Autodesk Inventor part; units mm, degrees
ref_plane "YZ Plane" through (0, 0, 0) normal (1, 0, 0) x (0, 1, 0)
ref_plane "XZ Plane" through (0, 0, 0) normal (0, 1, 0) x (-1, 0, 0)
ref_plane "XY Plane" through (0, 0, 0) normal (0, 0, 1) x (1, 0, 0)
sketch "Sketch1" plane through (0, 0, 0) normal (0, 1, 0) x (-1, 0, 0)
  circle A0 centre (0, 0) radius 2
  dimension "d0" = 4
extrude "Extrusion1" add sketch "Sketch1" along normal blind 12.506
sketch "Sketch2" plane through (0, 12.506, 0) normal (0, 1, 0) x (1, 0, 0)
  circle A0 centre (0, 0) radius 3
  dimension "d3" = 6
extrude "Extrusion2" add sketch "Sketch2" along normal blind 2.445
sketch "Sketch3" plane through (0, 14.951, 0) normal (0, 1, 0) x (1, 0, 0)
  circle A0 centre (0, 0) radius 2
  line L0 (0, 2) -> (1.7321, 1)
  line L1 (1.7321, 1) -> (1.7321, -1)
  line L2 (1.7321, -1) -> (0, -2)
  line L3 (0, -2) -> (-1.7321, -1)
  line L4 (-1.7321, -1) -> (-1.7321, 1)
  line L5 (-1.7321, 1) -> (0, 2)
extrude "Extrusion3" cut sketch "Sketch3" against normal blind 1.5 contours L1 L2 L3 L4 L5 L0
thread "Thread1"
properties part number "4mm_0.5_Screw"
Geometry: final body of the model. Coordinates: model frame, mm. A direction names the side the tool comes from. Coordinates: 2 decimals unless noted, no trailing zeros. Order: outer loops, then holes, each group sorted by start corner. A loop starts at its lowest first (then second) coordinate and runs counter-clockwise, first axis right, second up. Notation, with made-up numbers: M 66.5,82 L 90.5,82 A19 cw 90.5,111 Z; hole C 12.5,27.25 d4. An arc over 180 degrees is marked long. Answer in a Markdown table with one row per item. Add a question column.
Q1. Section query A-A on z = 0. Return the cut outline in (x, y), and give its area (3 significant figures).
Q2. Section query C-C on y = 10.25. Return the cut outline in (x, z).
Q3. Reachability of faces 1 (the flat face through (-0.88, 14.21, -1.49)), 2 (the flat face through (2, 14.951, 0)), 3 (the flat face through (1, 12.506, 2)) from +Z, -Z, +X, -X, +Y, -Y: full face, straight path, thin tool, end or side. Return the list, or none.
Q4. Section query D-D on z = -2.2. Return the cut outline in (x, y), and give its area (3 significant figures).
Q5. Mould query, pull axis Z, two halves, no side actions, for faces 4 (the cylindrical face through (-3, 14, 0)), 5 (the flat face through (0, 0, 0)), 6 (the flat face through (0, 13.451, 0)). Classes: released by +Z, released by -Z, zero draft, split by the parting line, or undercut.
Q6. Contact query for flat-ended pins moving along their axis: P1, Ø2, axis at y = 5, z = 1.5, coming from the -X side; P2, Ø1, axis at x = 1.5, y = 6, coming from the +Z side. Output: stop coordinate, or through.
Q7. Line query: L1, parallel to Y at x = 0.9, z = 0; L2, parallel to Z at x = 0, y = 2; L3, parallel to Y at x = -2.8, z = 0. Output: solid intervals per line, ascending.
Q8. Section query B-B on x = -0.5. Return the cut outline in (y, z), and give its area (3 significant figures).
Completed:
| question | item | result |
|---|---|---|
| 1 | outline | M -3,12.51 L -2,12.51 L -2,0 L 2,0 L 2,12.51 L 3,12.51 L 3,14.95 L 1.73,14.95 L 1.73,13.45 L -1.73,13.45 L -1.73,14.95 L -3,14.95 Z |
| 1 | area | 59.5 mm2 |
| 2 | outline | C 0,0 d4 |
| 3 | face 1 | +Y |
| 3 | face 2 | +Z, -Z, +X, -X, +Y |
| 3 | face 3 | -Y |
| 4 | outline | M -2.04,12.51 L 2.04,12.51 L 2.04,14.95 L -2.04,14.95 Z |
| 4 | area | 9.97 mm2 |
| 5 | face 4 | split by the parting line |
| 5 | face 5 | zero draft |
| 5 | face 6 | undercut |
| 6 | P1 | stops at x = -1.94 |
| 6 | P2 | stops at z = 1.73 |
| 7 | L1 | y = 0 to 13.45 |
| 7 | L2 | z = -2 to 2 |
| 7 | L3 | y = 12.51 to 14.95 |
| 8 | outline | M 0,-1.94 L 12.51,-1.94 L 12.51,-2.96 L 14.95,-2.96 L 14.95,-1.71 L 13.45,-1.71 L 13.45,1.71 L 14.95,1.71 L 14.95,2.96 L 12.51,2.96 L 12.51,1.94 L 0,1.94 Z |
| 8 | area | 57.8 mm2 |
